Model file for the job. Use its own axes, mm. A direction names the side the tool comes from. Coordinates: 2 decimals unless noted, no trailing zeros. Order: outer loops, then holes, each group sorted by start corner. A loop starts at its lowest first (then second) coordinate and runs counter-clockwise, first axis right, second up. Notation, with made-up numbers: (-26.5, -17.5) -> (-22.5, -17.5) arc R8 ccw to (-22.5, -12.5) -> close; hole circle Ø1 at (37, -30.75). An arc over 180 degrees is marked (long way). Return JSON: item names as keys, results as strings. Group by question number.
1) Flat gauge pins, fed straight in: pin 1 (8 mm diameter, centred on x = -51, y = -67, fed in from -Z); pin 2 (14.5 mm diameter, centred on x = 16.5, y = -27, fed in from -Z) (3 decimals); pin 3 (3 mm diameter, centred on x = -0.5, z = 18, fed in from -Y); pin 4 (2 mm diameter, centred on x = -10.5, z = -5, fed in from -Y). Where does each tip first touch, or does it go through?
2) Probe line 1 (X direction, y = 9, z = 0); line 2 (X direction, y = -52.5, z = -0.5); line 3 (Y direction, x = -17.5, z = 17.5). List the from-to ranges inside material, lowest first.
3) Cut at B-B (x = -20.75). Write the cut outline in (y, z) (3 decimals), and give its area (3 significant figures).
4) Cut at A-A (z = 3.5). Write the cut outline in (x, y) (3 decimals), and give its area (3 significant figures).
5) Cut at D-D (z = 11). Write the cut outline in (x, y).
6) Cut at C-C (x = 20.75). Write the cut outline in (y, z) (3 decimals).
7) Pull direction Z, two halves, no side cores. Call faces 1 (the cylindrical face through (-18.856, 6.211, -0.249)), 2 (the flat face through (0, 12.25, -8)), 3 (the flat face through (0, 6, 17.075)): +Z half, -Z half, draft (parallel to the pull), parting line (faces both ways), or undercut.
8) Which spindle directions (+Z, -Z, +X, -X, +Y, -Y) get a long thin tool onto all of the face, cutting with end or side? Do faces 4 (the flat face through (18, -46, 6.955)), 5 (the flat face through (-51, -67, 0)), 6 (the flat face through (-24, -58.59, 16)), 7 (the flat face through (-56, -69, 6.955)), 8 (the flat face through (0, 6, 7.075)). Say none if no direction does.
from build123d import *

# Parameters (mm, degrees)
SKETCH_1_W           = 51.5
SKETCH_1_H           = 34.15
SKETCH_1_W_2         = 31.5
SKETCH_1_H_2         = 14.15
EXTRUDE_1_DEPTH      = 12.25
SKETCH_2_R           = 1.91
CUT_EXTRUDE_1_DEPTH  = 34.236736076
SKETCH_4_W           = 13
SKETCH_4_H           = 13.91
EXTRUDE_1_2_DEPTH    = 74.82
SKETCH_5_W           = 13.91
SKETCH_5_H           = 16.23
EXTRUDE_2_DEPTH      = 16
SKETCH_7_R           = 25.25
SKETCH_7_R_2         = 15.25
EXTRUDE_2_2_DEPTH    = 16.23
SKETCH_15_R          = 1.91
CUT_EXTRUDE_6_DEPTH  = 97.964478439
SKETCH_16_W          = 13.91
SKETCH_16_H          = 16.23
EXTRUDE_4_DEPTH      = 10
SKETCH_17_R          = 1.91
CUT_EXTRUDE_7_DEPTH  = 102.16913771
SKETCH_23_W          = 89.330713517
SKETCH_23_H          = 36.104783584
CUT_EXTRUDE_12_DEPTH = 57


with BuildPart() as part:
    # 草圖1 → Extrude 1 (new body)
    with BuildSketch(Plane(origin=(0, 0, 0), x_dir=(1, 0, 0), z_dir=(0, 1, 0))):
        Rectangle(SKETCH_1_W, SKETCH_1_H)
        Rectangle(SKETCH_1_W_2, SKETCH_1_H_2, mode=Mode.SUBTRACT)
    extrude(amount=EXTRUDE_1_DEPTH)

    # 草圖2 → 除料-伸長1 (cut, through all)
    with BuildSketch(Plane(origin=(0, 12.25, 0), x_dir=(1, 0, 0), z_dir=(0, 1, 0))):
        with Locations(Location((-20.75, 0, 0), (0, 0, 270))):
            Circle(SKETCH_2_R)
        with Locations(Location((20.75, 0, 0), (0, 0, 270))):
            Circle(SKETCH_2_R)
    extrude(amount=-CUT_EXTRUDE_1_DEPTH, mode=Mode.SUBTRACT)

    # 草圖4 → Extrude 1 2 (add)
    with BuildSketch(Plane.XZ):
        with Locations((19.25, 0)):
            Rectangle(SKETCH_4_W, SKETCH_4_H)
    extrude(amount=EXTRUDE_1_2_DEPTH)

    # 草圖5 → Extrude 2 (add)
    with BuildSketch(Plane.ZY.offset(-12.75)):
        with Locations((0, -66.705)):
            Rectangle(SKETCH_5_W, SKETCH_5_H)
    extrude(amount=EXTRUDE_2_DEPTH)

    # 草圖7 → Extrude 2 2 (add)
    with BuildSketch(Plane(origin=(3.626674765, -74.82, 0), x_dir=(1, 0, 0), z_dir=(0, -1, 0))):
        with Locations((-30.978154344, 0)):
            Circle(SKETCH_7_R)
        with Locations((-30.978154344, 0)):
            Circle(SKETCH_7_R_2, mode=Mode.SUBTRACT)
    extrude(amount=-EXTRUDE_2_2_DEPTH)

    # 草圖15 → 除料-伸長6 (cut, through all)
    with BuildSketch(Plane(origin=(0, 0, -6.955), x_dir=(-1, 0, 0), z_dir=(0, 0, -1))):
        with Locations((-4.835883248, -66.705)):
            Circle(SKETCH_15_R)
    extrude(amount=-CUT_EXTRUDE_6_DEPTH, mode=Mode.SUBTRACT)

    # 草圖16 → 填料-伸長4 (add)
    with BuildSketch(Plane(origin=(-60, 0, 0), x_dir=(0, 0, -1), z_dir=(1, 0, 0))):
        with Locations((0, -66.705)):
            Rectangle(SKETCH_16_W, SKETCH_16_H)
    extrude(amount=EXTRUDE_4_DEPTH)

    # 草圖17 → 除料-伸長7 (cut, through all)
    with BuildSketch(Plane(origin=(0, 0, -6.955), x_dir=(-1, 0, 0), z_dir=(0, 0, -1))):
        with Locations((55.812362827, -66.705)):
            Circle(SKETCH_17_R)
    extrude(amount=-CUT_EXTRUDE_7_DEPTH, mode=Mode.SUBTRACT)

    # 草圖23 → 除料-伸長12 (cut)
    with BuildSketch(Plane(origin=(0, -58.59, 0), x_dir=(1, 0, 0), z_dir=(0, 1, 0))):
        with Locations((-31.915356759, 18.052391792)):
            Rectangle(SKETCH_23_W, SKETCH_23_H)
    extrude(amount=-CUT_EXTRUDE_12_DEPTH, mode=Mode.SUBTRACT)


solid = part.part
Answers below:
{
 "1": {"pin 1": "stops at z = 0", "pin 2": "stops at z = -6.955", "pin 3": "stops at y = 0", "pin 4": "passes through"},
 "2": {"line 1": "x = -25.75 to -22.66, -18.84 to -15.75, 15.75 to 18.84, 22.66 to 25.75", "line 2": "x = 12.75 to 25.75", "line 3": "y = -74.82 to -58.59"},
 "3": {"outline": "(-74.82, 13.747) -> (-58.59, 13.747) -> (-58.59, 24.372) -> (-74.82, 24.372) -> close; (0, -17.075) -> (12.25, -17.075) -> (12.25, -1.91) -> (0, -1.91) -> close; (0, 1.91) -> (12.25, 1.91) -> (12.25, 17.075) -> (0, 17.075) -> close", "area": "544 mm^2"},
 "4": {"outline": "(-60, -74.82) -> (-42.194, -74.82) -> (-42.194, -58.59) -> (-60, -58.59) -> close; (-25.75, 0) -> (-15.75, 0) -> (-15.75, 12.25) -> (-25.75, 12.25) -> close; (-12.509, -74.82) -> (25.75, -74.82) -> (25.75, 12.25) -> (15.75, 12.25) -> (15.75, 0) -> (12.75, 0) -> (12.75, -58.59) -> (-12.509, -58.59) -> close; hole circle Ø3.82 at (-55.812, -66.705); hole circle Ø3.82 at (4.836, -66.705)", "area": "1,890 mm^2"},
 "5": {"outline": "(-50.08, -74.82) -> (-37.91, -74.82) -> (-37.91, -58.59) -> (-50.08, -58.59) -> close; (-25.75, 0) -> (25.75, 0) -> (25.75, 12.25) -> (-25.75, 12.25) -> close; (-16.79, -74.82) -> (-4.62, -74.82) -> (-4.62, -58.59) -> (-16.79, -58.59) -> close"},
 "6": {"outline": "(-74.82, -6.955) -> (0, -6.955) -> (0, -17.075) -> (12.25, -17.075) -> (12.25, -1.91) -> (0, -1.91) -> (0, 1.91) -> (12.25, 1.91) -> (12.25, 17.075) -> (0, 17.075) -> (0, 6.955) -> (-74.82, 6.955) -> close"},
 "7": {"face 1": "undercut", "face 2": "draft", "face 3": "+Z half"},
 "8": {"face 4": "+Z, +X, -Y", "face 5": "-Z, -X, +Y, -Y", "face 6": "+Z, -Z, -X", "face 7": "+Z, -X, +Y, -Y", "face 8": "+Y"}
}
